from build123d import *

# Parameters (mm, degrees)
F0_R     = 5.715
F1_DEPTH = 78.74
F3_D     = 8.89
F3_DEPTH = 38.1
F3_TIP   = 2.6708254516
F4_R     = 5.715


with BuildPart() as f1:
    # F0 (on Top) → F1 (new body)
    with BuildSketch(Plane.XY):
        Circle(F0_R)
    extrude(amount=F1_DEPTH)

    # F3
    with Locations(Plane.XY.offset(78.74)):
        with Locations((0, 0)):
            Hole(F3_D / 2, depth=F3_DEPTH)
            with Locations((0, 0, -(F3_DEPTH + F3_TIP / 2))):  # 118° drill point
                Cone(0, F3_D / 2, F3_TIP, mode=Mode.SUBTRACT)

    # F6: sweep along a path in F5
    with BuildLine(Plane.XZ) as f6_path:
        Line((0, 0), (0, -31.75))
        ThreePointArc((0, -31.75), (1.8598719395, -36.2401280605), (6.35, -38.1))
        Line((6.35, -38.1), (85.09, -38.1))
    # F4 (on face) → F6 (sweep)
    with BuildSketch(Plane(origin=(0, 0, 0), x_dir=(1, 0, 0), z_dir=(0, 0, -1))):
        Circle(F4_R)
    sweep(path=f6_path.line)


solid = f1.part
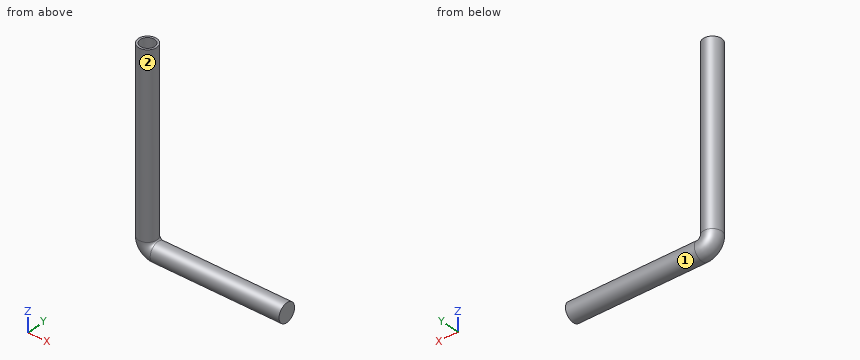
For this review, take the finished solid that the model builds, in its own axes (mm). Face numbers are marked on the shaded views. A direction names the side the tool comes from. Give positions to 0.01 mm unless a question says otherwise; leave off trailing zeros. Order: outer loops, then holes, each group sorted by start corner. A loop starts at its lowest first (then second) coordinate and runs counter-clockwise, first axis right, second up. Notation, with made-up numbers: M 21.5,-10.75 L 31.5,-10.75 A11 ccw 31.5,-3.75 Z; hole C 85,33 d9. An arc over 180 degrees is marked long. Answer in a Markdown table with one row per item. Add a question column.
(1) Wall thickness on probe 1 along X at (y, z) = (0, 59.5) (3 decimals); probe 2 along Z at (x, y) = (79, 0.5): over which ranges is each line inside the solid? List them lowest first. Write a range as [from, to].
(2) For the marked faces 1 and 2, list the 3-axis set-ups (+Z, -Z, +X, -X, +Y, -Y) from which the entire face can be reached by the end or side of a thin tool; tool diameter is ignored.
(3) Consider section C-C on x = 54. State the section outline as (y, z) points (3 decimals).
(4) Consider section B-B on z = 23. State the section outline as (x, y) points (3 decimals), and give its area (3 significant figures).
(5) For pin 1 (5 mm diameter, centred on x = 5.5, z = 23.5, fed in from +Y); pin 2 (2 mm diameter, centred on x = 58.5, y = 3, fed in from -Z); pin 3 (1 mm diameter, centred on y = -3.5, z = 18, fed in from -X), all flat-tipped, find the tip position at first contact; note any pin that passes through.
(6) Consider section A-A on z = 65. State the section outline as (x, y) points (3 decimals), and give its area (3 significant figures).
Evaluation:
| question | item | result |
|---|---|---|
| 1 | probe 1 | x = [-5.715, -4.445], [4.445, 5.715] |
| 1 | probe 2 | z = [-43.79, -32.41] |
| 2 | face 1 | +X |
| 2 | face 2 | +Z |
| 3 | outline | C 0,-38.1 d11.43 |
| 4 | outline | C 0,0 d11.43 |
| 4 | area | 103 mm^2 |
| 5 | pin 1 | stops at y = 4.86 |
| 5 | pin 2 | stops at z = -43.45 |
| 5 | pin 3 | stops at x = -4.86 |
| 6 | outline | C 0,0 d11.43; hole C 0,0 d8.89 |
| 6 | area | 40.5 mm^2 |
